from build123d import *

# Parameters (mm, degrees)
SKETCH2_R          = 2.38125
CUT_EXTRUDE1_DEPTH = 9
CIRPATTERN1_COUNT  = 2
CIRPATTERN1_ANGLE  = 120


with BuildPart() as part:
    # Sketch1 → Revolve1 (revolve)
    with BuildSketch(Plane.XY):
        Polygon((4, 0), (-4, 0), (-4, 9.652), (-2.222, 9.652), (-2.222, 10.287), (2.222, 10.287), (2.222, 9.652), (4, 9.652), align=None)
    revolve(axis=Axis((8.430806561, 0, 0), (-1, 0, 0)))

    # Sketch2 → Cut-Extrude1 (cut, through all)
    with BuildSketch(Plane.ZY.offset(4)):
        Circle(SKETCH2_R)
    extrude(amount=-CUT_EXTRUDE1_DEPTH, mode=Mode.SUBTRACT)

    # Sketch4 → #8-32 Tapped Hole1 (revolve, cut)
    with BuildSketch(Plane(origin=(0, 10.287, 0), x_dir=(0, 0, 1), z_dir=(1, 0, 0))):
        Polygon((0, 0), (0, 13.483806461), (1.7272, 12.446), (1.7272, 0), align=None)
    f_8_32_tapped_hole1 = revolve(axis=Axis((0, 16.637, 0), (0, -1, 0)), mode=Mode.SUBTRACT)

    # CirPattern1: #8-32 Tapped Hole1 ×2 about axis
    cirpattern1_axis = Axis((4, 0, 0), (-1, 0, 0))
    for i in range(1, CIRPATTERN1_COUNT):
        add(f_8_32_tapped_hole1.rotate(cirpattern1_axis, i * CIRPATTERN1_ANGLE / (CIRPATTERN1_COUNT - 1)), mode=Mode.SUBTRACT)


solid = part.part
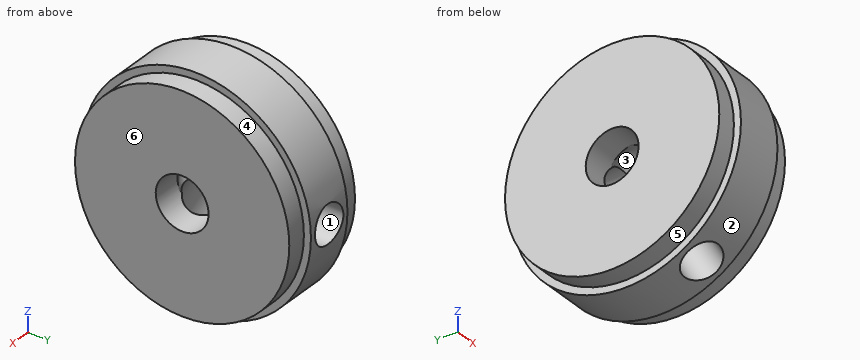
Part model, mm, in its own coordinate system. Face numbers are marked on the shaded views. A direction names the side the tool comes from. Give positions to 0.01 mm unless a question says otherwise; leave off trailing zeros. Loops run counter-clockwise (first coordinate to the right, second up) from the corner with the lowest first, then second, coordinate; pieces in that order, holes last. Notation, with made-up numbers: (75.25, -14) -> (101.25, -14) arc R20 cw to (101.25, 6) -> close; hole circle Ø11 at (-18.5, 13). An arc over 180 degrees is marked (long way). Write each question's results on one line, items separated by ' | '. Start each with the question number.
Q1. Which spindle directions (+Z, -Z, +X, -X, +Y, -Y) get a long thin tool onto all of the face, cutting with end or side? Do the marked faces 4, 5 and 6. Say none if no direction does.
Q2. Wall check: L1, parallel to Z at x = 3.5, y = 0; L2, parallel to Y at x = -1.25, z = -7; L3, parallel to Y at x = 1.75, z = -1.25. Give the ranges that are in metal, low to high.
Q3. Pin check, flat tips, straight feed: P1, Ø4, axis at x = 0, z = 0, coming from the +Y side; P2, Ø1, axis at x = 0.5, y = 6.5, coming from the -Z side; P3, Ø4, axis at x = -2, z = -4.5, coming from the +Y side. Stop position of each tip, or through.
Q4. Band-saw the part on A-A on y = 6.5. List the corners of the cut face in (x, z).
Q5. Band-saw the part on C-C on y = -7.75. List the corners of the cut face in (x, z).
Q6. Band-saw the part on D-D on z = 4. List the corners of the cut face in (x, y), plus the area to 3 significant figures.
Q7. Pull direction Y, two halves, no side cores. Call the marked faces 1, 2 and 3: +Y half, -Y half, draft (parallel to the pull), parting line (faces both ways), or undercut.
Q8. Band-saw the part on B-B on x = -2.75. List the corners of the cut face in (y, z), plus the area to 3 significant figures.
Results are:
1) face 4: +X | face 5: -X | face 6: +Z, -Z, +X, +Y, -Y
2) L1: z = -9.65 to -2.38, 2.38 to 9.65 | L2: y = -7.54 to -5.42, -2.67 to 7.54 | L3: y = -10.21 to -2.03, 2.03 to 10.21
3) P1: stops at y = 10.29 | P2: stops at z = -8.36 | P3: stops at y = 9.98
4) outline: (-4, -7.14) -> (-2.22, -7.14) -> (-2.22, -7.97) -> (2.22, -7.97) -> (2.22, -7.14) -> (4, -7.14) -> (4, 7.14) -> (2.22, 7.14) -> (2.22, 7.97) -> (-2.22, 7.97) -> (-2.22, 7.14) -> (-4, 7.14) -> close; hole circle Ø3.45 at (0, 0)
5) outline: (-4, -5.75) -> (-2.22, -5.75) -> (-2.22, -6.76) -> (2.22, -6.76) -> (2.22, -5.75) -> (4, -5.75) -> (4, 5.75) -> (2.22, 5.75) -> (2.22, 6.76) -> (-2.22, 6.76) -> (-2.22, 5.75) -> (-4, 5.75) -> close
6) outline: (-4, -8.78) -> (-2.22, -8.78) -> (-2.22, -9.48) -> (2.22, -9.48) -> (2.22, -8.78) -> (4, -8.78) -> (4, 8.78) -> (2.22, 8.78) -> (2.22, 9.48) -> (-2.22, 9.48) -> (-2.22, 8.78) -> (-4, 8.78) -> close | area: 147 mm²
7) face 1: draft | face 2: parting line | face 3: undercut
8) outline: circle Ø19.3 at (0, 0); hole circle Ø4.76 at (0, 0) | area: 275 mm²
